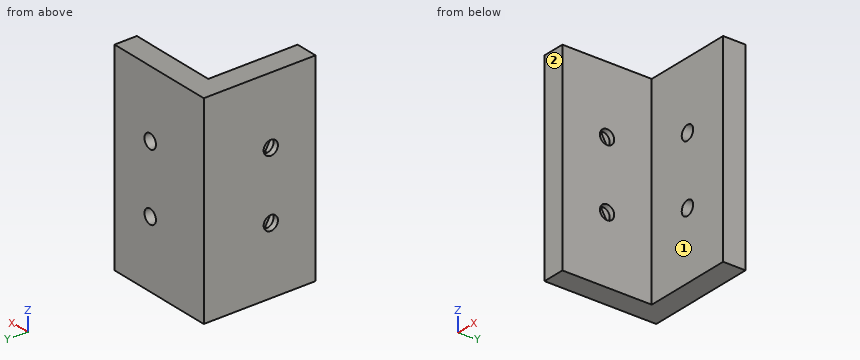
```python
from build123d import *

# Parameters (mm, degrees)
BOSS_EXTRUDE1_DEPTH = 45
CUT_EXTRUDE1_REACH  = 7
SKETCH2_R           = 1.6
CUT_EXTRUDE2_REACH  = 7
SKETCH3_R           = 1.6
CUT_EXTRUDE3_START  = -1.25
CUT_EXTRUDE3_DEPTH  = 2.5


with BuildPart() as part:
    # Sketch1 → Boss-Extrude1 (new body)
    with BuildSketch(Plane.XY):
        Polygon((0, 0), (0, -20), (-5, -20), (-5, 5), (20, 5), (20, 0), align=None)
    extrude(amount=BOSS_EXTRUDE1_DEPTH)

    # Sketch2 → Cut-Extrude1 (cut, up to next)
    with BuildSketch(Plane(origin=(0, 0, 0), x_dir=(0, 0, -1), z_dir=(1, 0, 0)), mode=Mode.PRIVATE) as cut_extrude1_sk1:
        with Locations((-30, -10)):
            Circle(SKETCH2_R)
    cut_extrude1_tool1 = extrude(cut_extrude1_sk1.sketch, amount=-CUT_EXTRUDE1_REACH, mode=Mode.PRIVATE) & part.part
    add(cut_extrude1_tool1.solids().sort_by_distance((0, -10, 30))[0], mode=Mode.SUBTRACT)
    # Sketch2 → Cut-Extrude1 (cut, up to next)
    with BuildSketch(Plane(origin=(0, 0, 0), x_dir=(0, 0, -1), z_dir=(1, 0, 0)), mode=Mode.PRIVATE) as cut_extrude1_sk2:
        with Locations((-15, -10)):
            Circle(SKETCH2_R)
    cut_extrude1_tool2 = extrude(cut_extrude1_sk2.sketch, amount=-CUT_EXTRUDE1_REACH, mode=Mode.PRIVATE) & part.part
    add(cut_extrude1_tool2.solids().sort_by_distance((0, -10, 15))[0], mode=Mode.SUBTRACT)

    # Sketch3 → Cut-Extrude2 (cut, up to next)
    with BuildSketch(Plane.XZ, mode=Mode.PRIVATE) as cut_extrude2_sk1:
        with Locations((10, 30)):
            Circle(SKETCH3_R)
    cut_extrude2_tool1 = extrude(cut_extrude2_sk1.sketch, amount=-CUT_EXTRUDE2_REACH, mode=Mode.PRIVATE) & part.part
    add(cut_extrude2_tool1.solids().sort_by_distance((10, 0, 30))[0], mode=Mode.SUBTRACT)
    # Sketch3 → Cut-Extrude2 (cut, up to next)
    with BuildSketch(Plane.XZ, mode=Mode.PRIVATE) as cut_extrude2_sk2:
        with Locations((10, 15)):
            Circle(SKETCH3_R)
    cut_extrude2_tool2 = extrude(cut_extrude2_sk2.sketch, amount=-CUT_EXTRUDE2_REACH, mode=Mode.PRIVATE) & part.part
    add(cut_extrude2_tool2.solids().sort_by_distance((10, 0, 15))[0], mode=Mode.SUBTRACT)

    # Sketch4 → Cut-Extrude3 (cut)
    with BuildSketch(Plane(origin=(0, 0, 0), x_dir=(0, 0, -1), z_dir=(1, 0, 0)).offset(CUT_EXTRUDE3_START)):
        Polygon((-30, -6.564765898), (-32.975, -8.282382949), (-32.975, -11.717617051), (-30, -13.435234102), (-27.025, -11.717617051), (-27.025, -8.282382949), align=None)
        Polygon((-15, -6.564765898), (-17.975, -8.282382949), (-17.975, -11.717617051), (-15, -13.435234102), (-12.025, -11.717617051), (-12.025, -8.282382949), align=None)
    extrude(amount=-CUT_EXTRUDE3_DEPTH, mode=Mode.SUBTRACT)


solid = part.part
```
Source: CAD feature listing. Evaluate the final solid. Frame: model axes, mm. Face numbers are marked on the shaded views. A direction names the side the tool comes from. Coordinates: 2 decimals unless noted, no trailing zeros. Loops run counter-clockwise (first coordinate to the right, second up) from the corner with the lowest first, then second, coordinate; pieces in that order, holes last. Notation, with made-up numbers: (45.5, -1.5) -> (61.5, -1.5) arc R23 cw to (61.5, 33.5) -> close; hole circle Ø4 at (37.25, 52.5). An arc over 180 degrees is marked (long way). One line per item, written item: value. Start each with the question number.
Q1. Line query: line 1 along Y through (x, z) = (-0.8, 30); line 2 along Y through (x, z) = (3.5, 39); line 3 along X through (y, z) = (-6, 8). Output: solid intervals per line, ascending.
Q2. Section query D-D, the plane z = 6. Return the cut outline in (x, y), and give its area (3 significant figures).
Q3. Section query C-C, the plane x = 10. Return the cut outline in (y, z).
Q4. Contact query for flat-ended pins moving along their axis: P1, Ø12, axis at x = 6.5, z = 31, coming from the -Y side; P2, Ø6.5, axis at y = -9, z = 16, coming from the +X side. Output: stop coordinate, or through.
Q5. Set-up query: the marked faces 1 and 2. Return all of +Z, -Z, +X, -X, +Y, -Y with unobstructed straight access to the full face (end or side cutting, diameter ignored); none if empty.
Q6. Section query B-B, the plane y = -10. Return the cut outline in (x, z) (3 decimals).
Q7. Section query A-A, the plane x = -2.25. Return the cut outline in (y, z) (3 decimals).
Results:
1. line 1: -20 to -11.6, -8.4 to 5
1. line 2: 0 to 5
1. line 3: -5 to 0
2. outline: (-5, -20) -> (0, -20) -> (0, 0) -> (20, 0) -> (20, 5) -> (-5, 5) -> close
2. area: 225 mm^2
3. outline: (0, 0) -> (5, 0) -> (5, 13.4) -> (0, 13.4) -> close; (0, 16.6) -> (5, 16.6) -> (5, 28.4) -> (0, 28.4) -> close; (0, 31.6) -> (5, 31.6) -> (5, 45) -> (0, 45) -> close
4. P1: y = 0
4. P2: x = 0
5. face 1: +Z, -Z, +X, -Y
5. face 2: +Z, -Z, +X, -X, -Y
6. outline: (-5, 0) -> (0, 0) -> (0, 13.4) -> (-1.25, 13.4) -> (-1.25, 12.025) -> (-3.75, 12.025) -> (-3.75, 13.4) -> (-5, 13.4) -> close; (-5, 16.6) -> (-3.75, 16.6) -> (-3.75, 17.975) -> (-1.25, 17.975) -> (-1.25, 16.6) -> (0, 16.6) -> (0, 28.4) -> (-1.25, 28.4) -> (-1.25, 27.025) -> (-3.75, 27.025) -> (-3.75, 28.4) -> (-5, 28.4) -> close; (-5, 31.6) -> (-3.75, 31.6) -> (-3.75, 32.975) -> (-1.25, 32.975) -> (-1.25, 31.6) -> (0, 31.6) -> (0, 45) -> (-5, 45) -> close
7. outline: (-20, 0) -> (5, 0) -> (5, 45) -> (-20, 45) -> close; hole (-13.435, 15) -> (-11.718, 12.025) -> (-8.282, 12.025) -> (-6.565, 15) -> (-8.282, 17.975) -> (-11.718, 17.975) -> close; hole (-13.435, 30) -> (-11.718, 27.025) -> (-8.282, 27.025) -> (-6.565, 30) -> (-8.282, 32.975) -> (-11.718, 32.975) -> close
